Autodesk Fusion 360 part; units mm, degrees
sketch "Sketch1" plane through (0, 0, 0) normal (0, 1, 0) x (1, 0, 0) in component "Nut_template"
  line L0 (0, 0) -> (101.6, 0)
  line L1 (101.6, 0) -> (101.6, -203.2)
  line L2 (101.6, -203.2) -> (0, -203.2)
  line L3 (0, -203.2) -> (0, 0)
  circle A0 centre (50.8, -101.6) radius 31.75
  line L4 (0, -203.2) -> (101.6, 0) construction
  line L5 (0, 0) -> (101.6, -203.2) construction
  point P0 (50.8, -101.6)
  dimension "d38" = 101.6
  dimension "d39" = 203.2
  dimension "d40" = 63.5
extrude "Extrude1" add sketch "Sketch1" along normal blind 63.5 in component "Nut_template"
thread "Thread1" in component "Nut_template"
component "Nut_template" placed x (1, 0, 0) y (0, 1, 0) z (0, 0, 1) at (0, 0, 0)
equation "d38 = nut_width"
equation "d39 = nut_length"
equation "d40 = screw_diameter"
equation "d41 = nut_thickness"
equation "screw_diameter = 2.5 in"
equation "nut_thickness = 2.5 in"
equation "nut_length = 8 in"
equation "nut_width = 4 in"
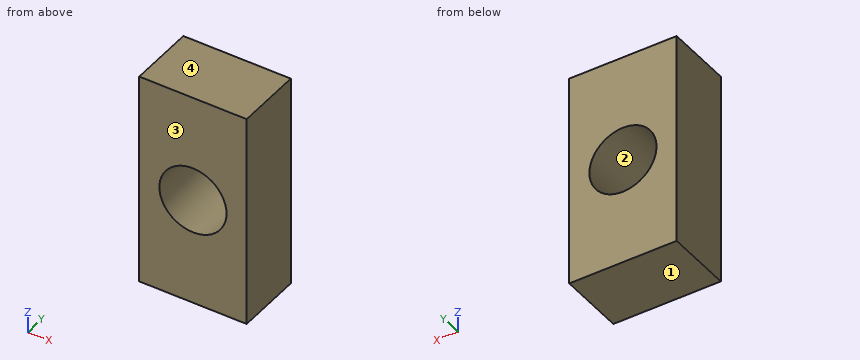
Input: part model. Units: mm. Frame: model coordinates. Face numbers are marked on the shaded views. Give positions to 0.01 mm unless a question says otherwise; leave off trailing zeros. Order: outer loops, then holes, each group sorted by start corner. A loop starts at its lowest first (then second) coordinate and runs counter-clockwise, first axis right, second up. Notation, with made-up numbers: (-27, 40.5) -> (26, 40.5) arc R14 ccw to (26, 53.5) -> close; hole circle Ø6 at (-26.75, 24.5). An arc over 180 degrees is marked (long way). Write each question's results on one line, items separated by ' | '. Start each with the question number.
Item 1: Mould query, pull axis Z, two halves, no side actions, for the marked faces 1, 2, 3 and 4. Classes: pulls with the +Z half, pulls with the -Z half, needs draft (parallel to the pull), parting line crosses it, or undercut.
Item 2: Cut plane A-A on x = 50.8. Return the cut outline in (y, z).
Item 3: Line query: line 1 (X direction, y = 50, z = 101); line 2 (Z direction, x = 50, y = 47); line 3 (Z direction, x = 57.5, y = 12). Output: solid intervals per line, ascending.
Item 4: Contact query for a flat-ended pin moving along its axis: P1, Ø6, axis at x = 56, z = 172, coming from the -Y side. Output: stop coordinate, or through.
Item 5: Cut plane C-C on y = 34. Return the cut outline in (x, z).
Item 6: Cut plane B-B on z = 101.6. Return the cut outline in (x, y), then the cut area to 3 significant figures.
Established:
1) face 1: pulls with the -Z half | face 2: undercut | face 3: needs draft | face 4: pulls with the +Z half
2) outline: (0, 0) -> (63.5, 0) -> (63.5, 69.85) -> (0, 69.85) -> close; (0, 133.35) -> (63.5, 133.35) -> (63.5, 203.2) -> (0, 203.2) -> close
3) line 1: 0 to 19.06, 82.54 to 101.6 | line 2: 0 to 69.86, 133.34 to 203.2 | line 3: 0 to 70.56, 132.64 to 203.2
4) P1: y = 0
5) outline: (0, 0) -> (101.6, 0) -> (101.6, 203.2) -> (0, 203.2) -> close; hole circle Ø63.5 at (50.8, 101.6)
6) outline: (0, 0) -> (19.05, 0) -> (19.05, 63.5) -> (0, 63.5) -> close; (82.55, 0) -> (101.6, 0) -> (101.6, 63.5) -> (82.55, 63.5) -> close | area: 2,420 mm^2
